from build123d import *

# Parameters (mm, degrees)
ESQUISSE1_R        = 1.5
BOSS_EXTRU_1_DEPTH = 5
CONG_1_R           = 6
CONG_2_R           = 3


with BuildPart() as part:
    # Esquisse1 → Boss.-Extru.1 (new body)
    with BuildSketch(Plane.XY):
        with BuildLine():
            Line((20, -3), (34, -3))
            Line((34, -3), (34, 8))
            Line((34, 8), (15, 8))
            ThreePointArc((15, 8), (7, 0), (15, -8))
            Line((15, -8), (20, -8))
            Line((20, -8), (20, -3))
        make_face()
        with Locations((15, 0)):
            Circle(ESQUISSE1_R, mode=Mode.SUBTRACT)
        with Locations((30, 0)):
            Circle(ESQUISSE1_R, mode=Mode.SUBTRACT)
    extrude(amount=BOSS_EXTRU_1_DEPTH)

    # Congé1
    # the kernel refuses this fillet: 6 mm, written as the material it adds along each edge
    with BuildSketch(Plane(origin=(20, -3, 0), x_dir=(-2.958065230920737e-05, -0.9999999995624925, 0), z_dir=(0, 0, 1))) as cong_1_piece_1:
        with BuildLine():
            CenterArc((5.999675, 5.916130485), CONG_1_R, 180.001694847, 80.407142396)
            Line((-0.000324998, 5.915953002), (-0.120324998, 5.915949452))
            ThreePointArc((-0.120324998, 5.915949452), (-0.120087499, 2.957972953), (-0.12, -3.55e-06))
            Line((-0.12, -3.55e-06), (3.55e-06, -0.12))
            ThreePointArc((3.55e-06, -0.12), (2.49999105, -0.119926049), (4.979981005, -0.11832261))
            Line((4.979981005, -0.11832261), (4.999975005, 0))
        make_face()
    extrude(amount=5)
    # the kernel refuses this fillet: 6 mm, written as the material it takes off along each edge
    with BuildSketch(Plane(origin=(34, 8, -14.999625005), x_dir=(-0.9999999996874845, 2.500062500775405e-05, 0), z_dir=(0, 0, 1))) as cong_1_2_piece_1:
        with BuildLine():
            CenterArc((5.999699998, 5.999999998), CONG_1_R, 180.00143243, 90)
            Line((-0.0003, 5.999849994), (-0.1203, 5.999846994))
            ThreePointArc((-0.1203, 5.999846994), (-0.120075, 2.999921999), (-0.12, -3e-06))
            Line((-0.12, -3e-06), (3e-06, -0.12))
            ThreePointArc((3e-06, -0.12), (2.999927999, -0.119925), (5.999853002, -0.12))
            Line((5.999853002, -0.12), (5.999850002, 0))
        make_face()
    extrude(amount=34.999250009, mode=Mode.SUBTRACT)
    with BuildSketch(Plane(origin=(20, -22.789882526, 5), x_dir=(2.9580652309207366e-05, 0, -0.9999999995624925), z_dir=(0, 1, 0))) as cong_1_2_piece_2:
        with BuildLine():
            CenterArc((5.999675, 5.916130485), CONG_1_R, 180.001694847, 80.407142396)
            Line((-0.000324998, 5.915953002), (-0.120324998, 5.915949452))
            ThreePointArc((-0.120324998, 5.915949452), (-0.120087499, 2.957972953), (-0.12, -3.55e-06))
            Line((-0.12, -3.55e-06), (3.55e-06, -0.12))
            ThreePointArc((3.55e-06, -0.12), (2.49999105, -0.119926049), (4.979981005, -0.11832261))
            Line((4.979981005, -0.11832261), (4.999975005, 0))
        make_face()
    extrude(amount=29.580664771, mode=Mode.SUBTRACT)
    with BuildSketch(Plane(origin=(20, -22.789882526, 0), x_dir=(2.9580652309207366e-05, 0, 0.9999999995624925), z_dir=(0, 1, 0))) as cong_1_2_piece_3:
        with BuildLine():
            CenterArc((5.999675, -5.916130485), CONG_1_R, 99.591162758, 80.407142396)
            Line((-0.000324998, -5.915953002), (-0.120324998, -5.915949452))
            ThreePointArc((-0.120324998, -5.915949452), (-0.120087499, -2.957972953), (-0.12, 3.55e-06))
            Line((-0.12, 3.55e-06), (3.55e-06, 0.12))
            ThreePointArc((3.55e-06, 0.12), (2.49999105, 0.119926049), (4.979981005, 0.11832261))
            Line((4.979981005, 0.11832261), (4.999975005, 0))
        make_face()
    extrude(amount=29.580664771, mode=Mode.SUBTRACT)

    # Congé2
    cong_2_edges = [part.edges().sort_by_distance(p)[0] for p in [
        (34, -3, 2.5),
    ]]
    fillet(cong_2_edges, radius=CONG_2_R)


solid = part.part
Build history of the part. All positions in model axes, mm. A direction names the side the tool comes from. Give positions to 0.01 mm unless a question says otherwise; leave off trailing zeros. Loops run counter-clockwise (first coordinate to the right, second up) from the corner with the lowest first, then second, coordinate; pieces in that order, holes last. Notation, with made-up numbers: (22.25, -25) -> (72.25, -25) arc R34 ccw to (72.25, 10) -> close; hole circle Ø10 at (-39.75, -24). An arc over 180 degrees is marked (long way). Answer in a Markdown table with one row per item.
Item 1: Mould opens along X. For faces 3 (the cylindrical face through (22.072, -4.393, 2.465)), 4 (the cylindrical face through (28.5, 0.07, 2.46)), 5 (the flat face through (17, -8, 2)) say: pulls with the +X half, pulls with the -X half, needs draft (parallel to the pull), parting line crosses it, or undercut.
Findings below:
| item | result |
|---|---|
| face 3 | pulls with the +X half |
| face 4 | undercut |
| face 5 | needs draft |
Item 2: Probe line 1 along Y through (x, z) = (15, 3.2); line 2 along X through (y, z) = (0.5, 4.35); line 3 along X through (y, z) = (0.25, 1.8). List the from-to ranges inside material, lowest first. Write a range as [from, to].
Findings below:
| item | result |
|---|---|
| line 1 | y = [-8, -1.5], [1.5, 8] |
| line 2 | x = [7.02, 13.59], [16.41, 28.59], [31.41, 34] |
| line 3 | x = [7, 13.52], [16.48, 28.52], [31.48, 34] |
Item 3: Slice it at A-A on z = 2.25. Give the number of separate pieces and of enclosed holes in the cut face, plus the area to 3 significant figures.
Findings below:
| item | result |
|---|---|
| separate pieces | 1 |
| enclosed holes | 2 |
| area | 318 mm² |
Item 4: Slice it at B-B on x = 29. Write the cut outline in (y, z), plus the area to 3 significant figures.
Findings below:
| item | result |
|---|---|
| outline | (-3, 0) -> (-1.12, 0) -> (-1.12, 5) -> (-3, 5) -> close; (1.12, 0) -> (7.92, 0) -> (7.92, 5) -> (1.12, 5) -> close |
| area | 43.4 mm² |
Item 5: Slice it at C-C on y = -0.75. Write the cut outline in (x, z).
Findings below:
| item | result |
|---|---|
| outline | (7.04, 0) -> (13.7, 0) -> (13.7, 5) -> (7.04, 5) -> close; (16.3, 0) -> (28.7, 0) -> (28.7, 5) -> (16.3, 5) -> close; (31.3, 0) -> (33.9, 0) -> (33.9, 5) -> (31.3, 5) -> close |
Item 6: Slice it at D-D on x = 21.25. Write the cut outline in (y, z), plus the area to 3 significant figures.
Findings below:
| item | result |
|---|---|
| outline | (-5.23, 0) -> (8, 0) -> (8, 5) -> (-5.23, 5) -> close |
| area | 66.1 mm² |
Item 7: Tool access for faces 1 (the flat face through (28, -3, 2)), 2 (the cylindrical face through (32.289, 6.196, 2.465)): list every direction of +Z, -Z, +X, -X, +Y, -Y with a clear straight run to the whole face (end or side of a thin tool).
Findings below:
| item | result |
|---|---|
| face 1 | +Z, -Z, +X, -Y |
| face 2 | +Z, -Z, +X, +Y |
Item 8: Flat gauge pins, fed straight in: P1, Ø2.5, axis at x = 30, y = 0, coming from the +Z side; P2, Ø3.5, axis at x = 15, y = 0, coming from the +Z side; P3, Ø1, axis at y = -4.5, z = 3, coming from the -X side; P4, Ø2.5, axis at x = 29.5, z = 2.5, coming from the -Y side. Where does each tip first touch, or does it go through?
Findings below:
| item | result |
|---|---|
| P1 | passes through |
| P2 | stops at z = 5 |
| P3 | stops at x = 8.07 |
| P4 | stops at y = -3 |
